Build history of the part. All positions in model axes, mm. A direction names the side the tool comes from. Give positions to 0.01 mm unless a question says otherwise; leave off trailing zeros. Loops run counter-clockwise (first coordinate to the right, second up) from the corner with the lowest first, then second, coordinate; pieces in that order, holes last. Notation, with made-up numbers: (-30.5, 44.5) -> (-7.5, 44.5) arc R30 cw to (-7.5, 79.5) -> close; hole circle Ø8 at (11.25, 31.25). An arc over 180 degrees is marked (long way). Answer as a JSON object with one key per item and string values. Group by question number.
from build123d import *

# Parameters (mm, degrees)
F0_W     = 50
F0_H     = 53.0426052851
F1_DEPTH = 50
F2_R     = 25
F3_DEPTH = 25
F4_DEPTH = 25
F5_T     = 2.5
F6_R     = 12.5
F7_DEPTH = 50


# Not quite as in the source:
# - a shell that OpenCascade refuses in one call is made with other operations: the cavity is built on its own and cut out


with BuildPart() as f1:
    # F0 (on Front) → F1 (new body)
    with BuildSketch(Plane.XZ):
        Rectangle(F0_W, F0_H)
    extrude(amount=-F1_DEPTH)

    # F2 (on Right) → F3 (cut)
    with BuildSketch(Plane.YZ):
        with Locations((-0.3665760159, -0.021956861)):
            Circle(F2_R)
    extrude(amount=F3_DEPTH, mode=Mode.SUBTRACT)

    # F2 (on Right) → F4 (cut)
    with BuildSketch(Plane.YZ):
        with Locations((-0.3665760159, -0.021956861)):
            Circle(F2_R)
    extrude(amount=-F4_DEPTH, mode=Mode.SUBTRACT)

    # F5: shell of thickness 2.5, made by hand


with BuildPart() as f5_core1:
    # F5_t2: copy of F1
    add(f1.part)

    # the walls: a layer under each face that stays
    f5_faces = [f5_core1.faces().sort_by_distance(p)[0] for p in [
        (-25, 25, 0),
        (25, 25, 0),
        (0, 0, -25.7702858998),
        (0, 25, -26.5213026426),
        (0, 50, 0),
        (0, 25, 26.5213026426),
        (0, 0, 25.7483290388),
    ]]
    thicken(f5_faces, amount=-F5_T, mode=Mode.SUBTRACT)


with BuildPart() as f1_1:
    add(f1.part)

    # what is left inside the walls is the cavity
    f5_cavity = [f5_core1.part.solids().sort_by_distance(p)[0] for p in [
        (-7.5, 24.658298, 0.057376),
    ]]
    add(f5_cavity, mode=Mode.SUBTRACT)

    # F6 (on Front) → F7 (cut)
    with BuildSketch(Plane.XZ):
        Circle(F6_R)
    extrude(amount=-F7_DEPTH, mode=Mode.SUBTRACT)


solid = f1_1.part
(1) 3-axis set-ups, long thin cutter, end or side, ignore diameter. For faces 4 (the flat face through (0, 27, -24.021)), 5 (the flat face through (0, 0, 26)): which of +Z, -Z, +X, -X, +Y, -Y reach the whole face in a straight line?
(2) Probe line 1 along Z through (x, y) = (2, 36); line 2 along Z through (x, y) = (0, 48.45); line 3 along X through (y, z) = (26, -6). List the from-to ranges inside material, lowest first. Write a range as [from, to].
(3) Pull direction X, two halves, no side cores. Call faces 1 (the flat face through (22.5, 31, 0)), 2 (the flat face through (25, 36, 0)), 3 (the flat face through (-11.5, 50, -5.5)): pulls with the +X half, pulls with the -X half, needs draft (parallel to the pull), parting line crosses it, or undercut.
(4) Pin check, flat tips, straight feed: pin 1 (4 mm diameter, centred on y = 19.5, z = 14.5, fed in from -X); pin 2 (6 mm diameter, centred on x = 15.5, z = 17, fed in from -Y). Stop position of each tip, or through.
(5) Saw through at D-D on x = -21.5. List the corners of the cut face in (y, z), plus the area to 3 significant figures.
(6) Saw through at C-C on z = 0. List the corners of the cut face in (x, y).
(7) Saw through at B-B on y = 41.5. List the corners of the cut face in (x, z).
(8) Saw through at A-A on x = 0. List the corners of the cut face in (y, z), plus the area to 3 significant figures.
Calculated:
{
 "1": {"face 4": "-Y", "face 5": "+Z, -Z, +X, -X, -Y"},
 "2": {"line 1": "z = [-26.52, -24.02], [24.02, 26.52]", "line 2": "z = [-26.52, -12.5], [12.5, 26.52]", "line 3": "x = [-25, -22.5], [22.5, 25]"},
 "3": {"face 1": "undercut", "face 2": "pulls with the +X half", "face 3": "needs draft"},
 "4": {"pin 1": "stops at x = -25", "pin 2": "stops at y = 47.5"},
 "5": {"outline": "(0, -26.52) -> (50, -26.52) -> (50, 26.52) -> (0, 26.52) -> (0, 24.98) arc R25 cw to (6.48, 24.02) -> (47.5, 24.02) -> (47.5, -24.02) -> (6.64, -24.02) arc R25 cw to (0, -25.02) -> close", "area": "362 mm^2"},
 "6": {"outline": "(-25, 24.63) -> (-22.5, 24.63) -> (-22.5, 47.5) -> (-12.5, 47.5) -> (-12.5, 50) -> (-25, 50) -> close; (12.5, 47.5) -> (22.5, 47.5) -> (22.5, 24.63) -> (25, 24.63) -> (25, 50) -> (12.5, 50) -> close"},
 "7": {"outline": "(-25, -26.52) -> (25, -26.52) -> (25, 26.52) -> (-25, 26.52) -> close; hole (-22.5, -24.02) -> (22.5, -24.02) -> (22.5, 24.02) -> (-22.5, 24.02) -> close"},
 "8": {"outline": "(0, -26.52) -> (50, -26.52) -> (50, -12.5) -> (47.5, -12.5) -> (47.5, -24.02) -> (6.64, -24.02) arc R25 cw to (0, -25.02) -> close; (0, 24.98) arc R25 cw to (6.48, 24.02) -> (47.5, 24.02) -> (47.5, 12.5) -> (50, 12.5) -> (50, 26.52) -> (0, 26.52) -> close", "area": "299 mm^2"}
}
